Autodesk Inventor part; units mm, degrees
ref_plane "YZ Plane" through (0, 0, 0) normal (1, 0, 0) x (0, 1, 0)
ref_plane "XZ Plane" through (0, 0, 0) normal (0, 1, 0) x (-1, 0, 0)
ref_plane "XY Plane" through (0, 0, 0) normal (0, 0, 1) x (1, 0, 0)
sketch "Sketch1" plane through (0, 0, 0) normal (0, 1, 0) x (-1, 0, 0)
  line L0 (0, 0) -> (42.0116, 0)
  line L1 (42.0116, 0) -> (42.0116, -59.0296)
  line L2 (42.0116, -59.0296) -> (0, -59.0296)
  line L3 (0, -59.0296) -> (0, 0)
  dimension "d0" = 42.0116
  dimension "d1" = 59.0296
extrude "Plate1" add sketch "Sketch1" along normal blind 1.5875
sketch "Sketch2" plane through (-42.0116, 1.5875, 0) normal (-1, 0, 0) x (0, -1, 0)
  line L0 (0, -59.0296) -> (0, 0)
  line L1 (0, 0) -> (-94.6023, 0)
  line L2 (-94.6023, 0) -> (-94.6023, -59.0296)
  line L3 (-94.6023, -59.0296) -> (0, -59.0296)
edge flange "Flange1" height 96.1898 angle 90 thickness 1.5875 bend radius 1.5875 thickness toward (-1, 0, 0) relief straight relief width 1.5875 relief depth 0.7937 corner gap 1.5875 corner form 0 edges at (-42.0116, 1.5875, -29.5148) (0, 1.5875, -29.5148) wall of the first edge with corners at (-42.0116, 1.5875, -59.0296) (-42.0116, 1.5875, 0) (-42.0116, 96.1898, 0) (-42.0116, 96.1898, -59.0296)
bend "Bend1"
corner "Corner1"
sketch "Sketch3" plane through (1.5875, 96.1898, 0) normal (1, 0, 0) x (0, 0, -1)
  circle A0 centre (4.0046, -7.3) radius 2.0193
  circle A1 centre (48.836, -7.3) radius 2.0193
  circle A2 centre (48.836, -32.7) radius 2.0193
  circle A3 centre (48.836, -32.7) radius 2.0193
  circle A4 centre (4.0046, -32.7) radius 2.0193
  point P0 (0, -96.1898)
extrude "Extrusion1" cut sketch "Sketch3" against normal up to surface (45.1866 mm away)
equation "\"d3\" = BendReliefWidth"
equation "\"d4\" = BendReliefDepth"
equation "\"d5\" = MinimumRemnant"
equation "\"d6\" = BendRadius"
equation "\"d9\" = BendRadius"
equation "\"d10\" = CornerReliefSize"
equation "\"d11\" = GapSize"
equation "\"d12\" = JacobiRadiusSize"
equation "\"BendRadius\" = Thickness"
equation "\"BendReliefWidth\" = Thickness"
equation "\"BendReliefDepth\" = 0.5 * Thickness"
equation "\"CornerReliefSize\" = 4 * Thickness"
equation "\"MinimumRemnant\" = 2 * Thickness"
equation "\"TransitionRadius\" = BendRadius"
equation "\"JacobiRadiusSize\" = Thickness"
equation "\"GapSize\" = Thickness"
equation "\"d2\" = BendRadius"
properties part number "lifterMountB"
Build history of the part. All positions in model axes, mm. A direction names the side the tool comes from. Give positions to 0.01 mm unless a question says otherwise; leave off trailing zeros. Loops run counter-clockwise (first coordinate to the right, second up) from the corner with the lowest first, then second, coordinate; pieces in that order, holes last.
1) Band-saw the part on B-B on z = -3.5. State how many separate pieces and enclosed holes the cut face has, then the cut area to 3 significant figures.
Values follow:
separate pieces: 5
enclosed holes: 0
area: 344 mm2
2) 3-axis set-ups, long thin cutter, end or side, ignore diameter. For faces 1 (the face through (-42.794, 61.519, -3.567)), 2 (the face through (-42.012, 49, -29)): which of +Z, -Z, +X, -X, +Y, -Y reach the whole face in a straight line?
Values follow:
face 1: +X, -X
face 2: +Z, -Z, +Y
3) Probe line 1 along X through (y, z) = (67.5, -7.5); line 2 along Y through (x, z) = (-19, -32.5). List the from-to ranges inside material, lowest first.
Values follow:
line 1: x = -43.6 to -42.01, 0 to 1.59
line 2: y = 0 to 1.59
4) Band-saw the part on D-D on x = -30.5. List the corners of the cut face in (y, z).
Values follow:
outline: (0, -59.03) - (1.59, -59.03) - (1.59, 0) - (0, 0) - close
5) Band-saw the part on A-A on y = 51. List the corners of the cut face in (x, z).
Values follow:
outline: (-43.6, -59.03) - (-42.01, -59.03) - (-42.01, 0) - (-43.6, 0) - close; (0, -59.03) - (1.59, -59.03) - (1.59, 0) - (0, 0) - close
6) Drop flat-ended pins along their axis: P1, Ø2.5, axis at y = 88.89, z = -48.84, coming from the +X side; P2, Ø8, axis at x = -17.5, z = -30.5, coming from the +Y side. Give the stop position or say it passes through.
Values follow:
P1: passes through
P2: stops at y = 1.59
7) Two-plate mould, pull along Z, no slides. Class faces 3 (the face through (-42.79, 90.89, -48.57)), 4 (the face through (-21, 0, -29)), 5 (the face through (-43, 48, 0)): released by +Z, released by -Z, zero draft, split by the parting line, or undercut.
Values follow:
face 3: undercut
face 4: zero draft
face 5: released by +Z
